Geometry check sheet. Reference: the model listing, model coordinates, mm. A direction names the side the tool comes from. Round coordinates to 2 decimals unless told otherwise and drop trailing zeros. Write each loop counter-clockwise with the first axis right and the second up, starting at its lowest first coordinate (ties: lowest second). Pieces come first, ordered by that corner, then holes. Notation, with made-up numbers: (28, 48) -> (42, 48) arc R34 cw to (42, 82) -> close; hole circle Ø9 at (72.5, 80.25). An arc over 180 degrees is marked (long way). Use a Markdown table: item, result.
```python
from build123d import *

# Parameters (mm, degrees)
SKETCH_1_W          = 40
SKETCH_1_H          = 19.9
EXTRUDE_1_DEPTH     = 28
SKETCH_2_W          = 54
SKETCH_2_H          = 19.9
EXTRUDE_2_DEPTH     = 2
SKETCH_3_W          = 40
SKETCH_3_H          = 19.9
EXTRUDE_3_DEPTH     = 5
SKETCH_4_R          = 1.5
CUT_EXTRUDE_1_DEPTH = 42.569249452
SKETCH_5_R          = 3
EXTRUDE_4_DEPTH     = 6.5
SKETCH_7_R          = 6
EXTRUDE_5_DEPTH     = 3
SKETCH_8_R          = 4.5
EXTRUDE_6_DEPTH     = 2
SKETCH_9_R          = 10
EXTRUDE_7_DEPTH     = 2.5
SKETCH_10_R         = 1.5
CUT_EXTRUDE_2_DEPTH = 2.5
SKETCH_11_R         = 1.5
CUT_EXTRUDE_3_DEPTH = 6


with BuildPart() as part:
    # 草图1 → 凸台-拉伸1 (new body)
    with BuildSketch(Plane(origin=(0, 0, 0), x_dir=(1, 0, 0), z_dir=(0, 1, 0))):
        Rectangle(SKETCH_1_W, SKETCH_1_H)
    extrude(amount=EXTRUDE_1_DEPTH)

    # 草图2 → 凸台-拉伸2 (add)
    with BuildSketch(Plane(origin=(0, 28, 0), x_dir=(1, 0, 0), z_dir=(0, 1, 0))):
        Rectangle(SKETCH_2_W, SKETCH_2_H)
    extrude(amount=EXTRUDE_2_DEPTH)

    # 草图3 → 凸台-拉伸3 (add)
    with BuildSketch(Plane(origin=(0, 30, 0), x_dir=(1, 0, 0), z_dir=(0, 1, 0))):
        Rectangle(SKETCH_3_W, SKETCH_3_H)
    extrude(amount=EXTRUDE_3_DEPTH)

    # 草图4 → 切除-拉伸1 (cut, through all)
    with BuildSketch(Plane(origin=(0, 30, 0), x_dir=(1, 0, 0), z_dir=(0, 1, 0))):
        with Locations(Location((-24.3, 4.5, 0), (0, 0, 270))):
            Circle(SKETCH_4_R)
        with Locations(Location((24.3, 4.5, 0), (0, 0, 270))):
            Circle(SKETCH_4_R)
        with Locations(Location((24.3, -4.5, 0), (0, 0, 270))):
            Circle(SKETCH_4_R)
        with Locations(Location((-24.3, -4.5, 0), (0, 0, 270))):
            Circle(SKETCH_4_R)
    extrude(amount=-CUT_EXTRUDE_1_DEPTH, mode=Mode.SUBTRACT)

    # 草图5 → 凸台-拉伸4 (add)
    with BuildSketch(Plane(origin=(0, 35, 0), x_dir=(1, 0, 0), z_dir=(0, 1, 0))):
        with Locations(Location((10, 0, 0), (0, 0, 90))):
            Circle(SKETCH_5_R)
    extrude(amount=EXTRUDE_4_DEPTH)

    # 草图7 → 凸台-拉伸5 (add)
    with BuildSketch(Plane(origin=(0, 35, 0), x_dir=(1, 0, 0), z_dir=(0, 1, 0))):
        with Locations(Location((10, 0, 0), (0, 0, 90))):
            Circle(SKETCH_7_R)
    extrude(amount=EXTRUDE_5_DEPTH)

    # 草图8 → 凸台-拉伸6 (add)
    with BuildSketch(Plane(origin=(0, 41.5, 0), x_dir=(1, 0, 0), z_dir=(0, 1, 0))):
        with Locations(Location((10, 0, 0), (0, 0, 270))):
            Circle(SKETCH_8_R)
    extrude(amount=-EXTRUDE_6_DEPTH)

    # 草图9 → 凸台-拉伸7 (add)
    with BuildSketch(Plane(origin=(0, 41.5, 0), x_dir=(1, 0, 0), z_dir=(0, 1, 0))):
        with Locations(Location((10, 0, 0), (0, 0, 270))):
            Circle(SKETCH_9_R)
    extrude(amount=EXTRUDE_7_DEPTH)

    # 草图10 → 切除-拉伸2 (cut)
    with BuildSketch(Plane(origin=(0, 44, 0), x_dir=(1, 0, 0), z_dir=(0, 1, 0))):
        with Locations(Location((10, 7, 0), (0, 0, 270))):
            Circle(SKETCH_10_R)
        with Locations(Location((17, 0, 0), (0, 0, 270))):
            Circle(SKETCH_10_R)
        with Locations(Location((10, -7, 0), (0, 0, 270))):
            Circle(SKETCH_10_R)
        with Locations(Location((3, 0, 0), (0, 0, 270))):
            Circle(SKETCH_10_R)
    extrude(amount=-CUT_EXTRUDE_2_DEPTH, mode=Mode.SUBTRACT)

    # 草图11 → 切除-拉伸3 (cut)
    with BuildSketch(Plane(origin=(0, 44, 0), x_dir=(1, 0, 0), z_dir=(0, 1, 0))):
        with Locations(Location((10, 0, 0), (0, 0, 270))):
            Circle(SKETCH_11_R)
    extrude(amount=-CUT_EXTRUDE_3_DEPTH, mode=Mode.SUBTRACT)


solid = part.part
```
(1) Thickness scan on line 1 (X direction, y = 42.55, z = 0); line 2 (Y direction, x = 6.5, z = 4.5); line 3 (Y direction, x = 13.5, z = 7.75). Record the ranges inside material, lowest first.
A:
| item | result |
|---|---|
| line 1 | x = 0 to 1.5, 4.5 to 8.5, 11.5 to 15.5, 18.5 to 20 |
| line 2 | y = 0 to 38, 41.5 to 44 |
| line 3 | y = 0 to 35, 41.5 to 44 |
(2) Section check B-B on x = -24.3. Record the cut outline in (y, z), plus the area to 3 significant figures.
A:
| item | result |
|---|---|
| outline | (28, -9.95) -> (30, -9.95) -> (30, -6) -> (28, -6) -> close; (28, -3) -> (30, -3) -> (30, 3) -> (28, 3) -> close; (28, 6) -> (30, 6) -> (30, 9.95) -> (28, 9.95) -> close |
| area | 27.8 mm2 |
(3) Section check C-C on y = 40.5. Record the cut outline in (x, z).
A:
| item | result |
|---|---|
| outline | circle Ø9 at (10, 0); hole circle Ø3 at (10, 0) |
(4) Gauge pin test, flat ends, axial feed: pin 1 Ø1.5 at (x, z) = (10, 0.5) entering from +Y; pin 2 Ø6 at (y, z) = (12.5, -2) entering from -X; pin 3 Ø3 at (x, y) = (-8, 27) entering from -Z. Record the tip position at first contact, or that the pin passes through.
A:
| item | result |
|---|---|
| pin 1 | stops at y = 38 |
| pin 2 | stops at x = -20 |
| pin 3 | stops at z = -9.95 |
(5) Section check D-D on y = 21. Record the cut outline in (x, z), plus the area to 3 significant figures.
A:
| item | result |
|---|---|
| outline | (-20, -9.95) -> (20, -9.95) -> (20, 9.95) -> (-20, 9.95) -> close |
| area | 796 mm2 |
(6) Access from +Z, -Z, +X, -X, +Y, -Y to the whole of each face (thin tool, end or side, straight path). Record for faces 5 (the face through (15.323, 36.479, -2.769)), 6 (the face through (1.536, 42.768, -0.325)), 7 (the face through (-24, 28, 0)).
A:
| item | result |
|---|---|
| face 5 | none |
| face 6 | +Y |
| face 7 | +Z, -Z, -X, -Y |
(7) Release check for a two-part mould opening along X. For faces 1 (the face through (20, 32, 0)), 2 (the face through (10, 38, 0)), 3 (the face through (-20, 14, 0)), 4 (the face through (23, 28, 0)) record: +X half, -X half, draft (parallel to the pull), parting line (faces both ways), or undercut.
A:
| item | result |
|---|---|
| face 1 | +X half |
| face 2 | undercut |
| face 3 | -X half |
| face 4 | draft |
(8) Section check A-A on z = 7. Record the cut outline in (x, y).
A:
| item | result |
|---|---|
| outline | (-27, 28) -> (-20, 28) -> (-20, 0) -> (20, 0) -> (20, 28) -> (27, 28) -> (27, 30) -> (20, 30) -> (20, 35) -> (-20, 35) -> (-20, 30) -> (-27, 30) -> close; (2.86, 41.5) -> (8.5, 41.5) -> (8.5, 44) -> (2.86, 44) -> close; (11.5, 41.5) -> (17.14, 41.5) -> (17.14, 44) -> (11.5, 44) -> close |
